Design review of the part shown in the three views and the two pictorial views. Dimensions are in mm from the part's minimum x, y and z. A direction names the side the tool comes from. Coordinates: 2 decimals unless noted, no trailing zeros. Loops run counter-clockwise (first coordinate to the right, second up) from the corner with the lowest first, then second, coordinate; pieces in that order, holes last. Notation, with made-up numbers: (75.5, -27.5) -> (97.5, -27.5) arc R12 cw to (97.5, -13.5) -> close; hole circle Ø9 at (84, 55). An arc over 180 degrees is marked (long way). One line per item, written item: value. Start each with the question number.
1. Insertion check: pin 1 (0.6 mm diameter, centred on y = 6, z = 13, fed in from +X); pin 2 (5 mm diameter, centred on x = 1, z = 10.5, fed in from +Y); pin 3 (6 mm diameter, centred on x = 1.5, z = 8, fed in from -Y); pin 4 (1.5 mm diameter, centred on x = 8, y = 6, fed in from -Z). Each pin has a flat end and moves straight along its axis. Give the tip position at first contact, or say it passes through.
2. Add section A-A on x = 5. Write out the cut boundary in (y, z), plus the area to 3 significant figures.
3. Add section C-C on z = 12.25. Write out the cut boundary in (x, y), plus the area to 3 significant figures.
4. Machinability: for the marked faces 1 and 2, which of the approach directions +Z, -Z, +X, -X, +Y, -Y give a long, thin tool a straight path to every point of the face, cutting with its end or side? Answer none if there is none.
5. Add section B-B on y = 5. Write out the cut boundary in (x, z), plus the area to 3 significant figures.
6. Add section D-D on x = 7. Write out the cut boundary in (y, z).
7. For probe 1 along Z at (x, y) = (5.5, 0.75); probe 2 along Z at (x, y) = (5.25, 3.5); probe 3 along X at (y, z) = (1, 13), list the stretches that pass through material, from the lowest coordinate up.
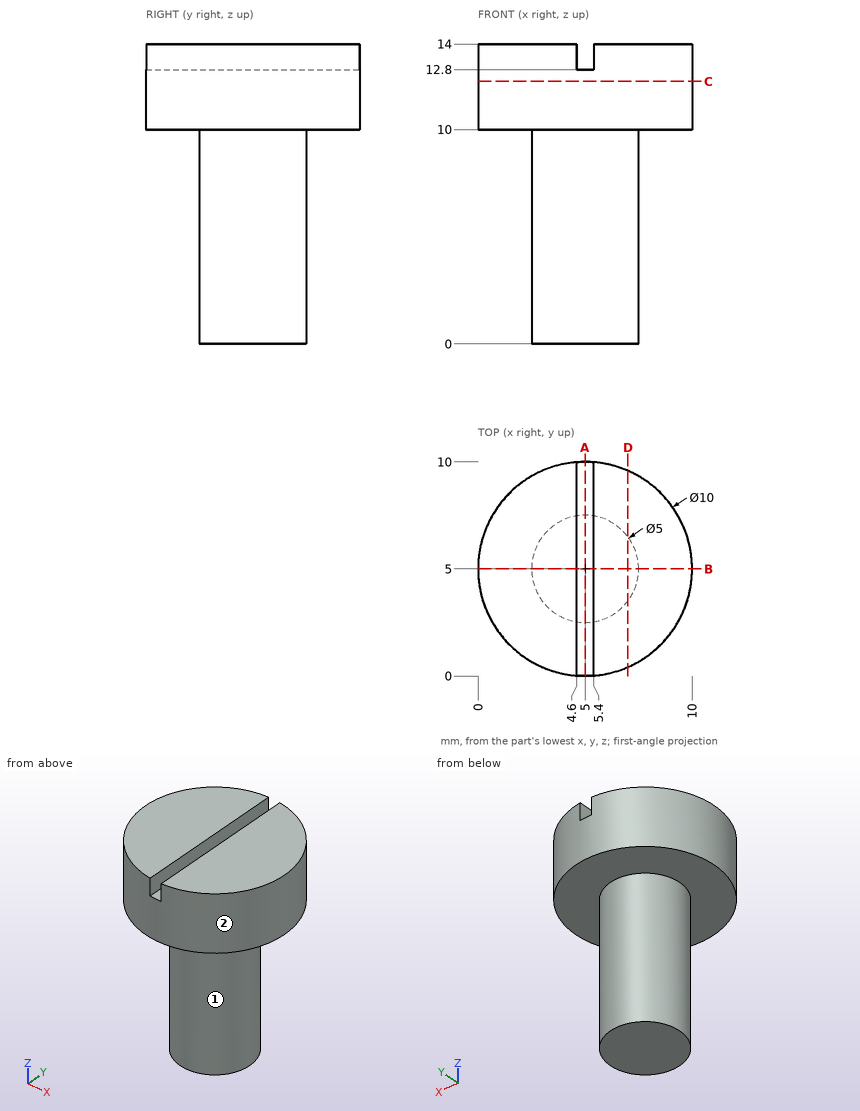
Worked answers:
1. pin 1: stops at x = 9.95
1. pin 2: stops at y = 9.77
1. pin 3: stops at y = 0.16
1. pin 4: stops at z = 0
2. outline: (0, 10) -> (2.5, 10) -> (2.5, 0) -> (7.5, 0) -> (7.5, 10) -> (10, 10) -> (10, 12.8) -> (0, 12.8) -> close
2. area: 78.0 mm²
3. outline: circle Ø10 at (5, 5)
3. area: 78.5 mm²
4. face 1: -Z
4. face 2: +Z, -Z
5. outline: (0, 10) -> (2.5, 10) -> (2.5, 0) -> (7.5, 0) -> (7.5, 10) -> (10, 10) -> (10, 14) -> (5.4, 14) -> (5.4, 12.8) -> (4.6, 12.8) -> (4.6, 14) -> (0, 14) -> close
5. area: 89.0 mm²
6. outline: (0.42, 10) -> (3.5, 10) -> (3.5, 0) -> (6.5, 0) -> (6.5, 10) -> (9.58, 10) -> (9.58, 14) -> (0.42, 14) -> close
7. probe 1: z = 10 to 14
7. probe 2: z = 0 to 12.8
7. probe 3: x = 2 to 4.6, 5.4 to 8
